```python
from build123d import *

# Parameters (mm, degrees)
F0_R     = 11.43
F2_R     = 8.89
F4_R     = 5.715
F5_DEPTH = 2.286
F6_R     = 0.508


with BuildPart() as f3:
    # F0 (on Top) → F3 section 0
    with BuildSketch(Plane.XY):
        Circle(F0_R)
    # F2 (on offset) → F3 section 1
    with BuildSketch(Plane.XY.offset(15.24)):
        Circle(F2_R)
    loft()

    # F4 (on face) → F5 (cut)
    with BuildSketch(Plane.XY.offset(15.24)):
        Circle(F4_R)
    extrude(amount=-F5_DEPTH, mode=Mode.SUBTRACT)

    # F6
    f6_edges = [f3.edges().sort_by_distance(p)[0] for p in [
        (-5.715, 0, 15.24),
        (-8.89, 0, 15.24),
    ]]
    fillet(f6_edges, radius=F6_R)


solid = f3.part
```
Could you check a few things on this model? Use its own coordinates, in mm. A direction names the side the tool comes from. Round coordinates to 2 decimals unless told otherwise and drop trailing zeros. Write each loop counter-clockwise with the first axis right and the second up, starting at its lowest first coordinate (ties: lowest second). Pieces come first, ordered by that corner, then holes. Notation, with made-up numbers: M -15,-13 L -7,-13 A26 ccw -7,8 Z; hole C -31,-30 d11. An arc over 180 degrees is marked long. Answer in a Markdown table with one row per item. Add a question column.
Q1. Imagine slicing it at C-C (z = 1.5). Please give me the cut outline in (x, y).
Q2. Imagine slicing it at A-A (x = 0). Please give me the cut outline in (y, z) (3 decimals).
Q3. If we mould it in two halves opening along Y, with no side actions, what happens to faces 3 (the cylindrical face through (5.45, 1.72, 13.86)), 4 (the flat face through (-5, 4, 15.24)), 5 (the conical face through (-7.859, -6.026, 9.158))? For each: +Y half, -Y half, draft (parallel to the pull), parting line (faces both ways), or undercut.
Q4. If I drill on line 1 (Y direction, x = 0, z = 13.9) (3 decimals); line 2 (Y direction, x = -3.25, z = 14); line 3 (Z direction, x = -1, y = 5.5), over which ranges is the centre line in solid material (lowest first)? Write a range as from..to.
Q5. Will these pins go through, and if not, where does the flat tip stop? pin 1 Ø1.5 at (x, z) = (1, 5.5) entering from +Y; pin 2 Ø1.5 at (x, z) = (7, 12.5) entering from -Y; pin 3 Ø4 at (x, z) = (4, 11) entering from -Y.
Q6. Imagine slicing it at B-B (z = 12). Please give me the cut outline in (x, y), then the cut area to 3 significant figures.
Q7. On a 3-axis mill with a long thin cutter (end or side, diameter ignored), from which of +Z, -Z, +X, -X, +Y, -Y can I reach the whole of each face in a straight line? I mean faces 1 (the flat face through (0, 0, 0)), 2 (the flat face through (0, 0, 12.954)). Say none if no direction works.
Values:
| question | item | result |
|---|---|---|
| 1 | outline | C 0,0 d22.36 |
| 2 | outline | M -11.43,0 L 11.43,0 L 8.961,14.816 A0.508 ccw 8.46,15.24 L 6.223,15.24 A0.508 ccw 5.715,14.732 L 5.715,12.954 L -5.715,12.954 L -5.715,14.732 A0.508 ccw -6.223,15.24 L -8.46,15.24 A0.508 ccw -8.961,14.816 Z |
| 3 | face 3 | undercut |
| 3 | face 4 | draft |
| 3 | face 5 | parting line |
| 4 | line 1 | -9.113..-5.715, 5.715..9.113 |
| 4 | line 2 | -8.5..-4.7, 4.7..8.5 |
| 4 | line 3 | 0..12.95 |
| 5 | pin 1 | y = 10.6 |
| 5 | pin 2 | y = -6.97 |
| 5 | pin 3 | y = -9.5 |
| 6 | outline | C 0,0 d18.86 |
| 6 | area | 279 mm^2 |
| 7 | face 1 | -Z, +X, -X, +Y, -Y |
| 7 | face 2 | +Z |
